Verification items for the finished model (mm, model axes). A direction names the side the tool comes from. Give positions to 0.01 mm unless a question says otherwise; leave off trailing zeros. Write each question's results on one line, items separated by ' | '. Start each with the question number.
1. Material ranges on L1, parallel to Y at x = -57, z = 0.8; L2, parallel to Y at x = 64.5, z = 0.55; L3, parallel to Y at x = -56, z = 0.8, recorded low to high. Write a range as from..to.
2. Cross-section at A-A, the plane z = 0.8. State how many separate pieces and enclosed holes the cut face has, then the cut area to 3 significant figures.
3. Depth check by flat-ended pin: pin 1 Ø0.6 at (y, z) = (5, 0.5) entering from +X; pin 2 Ø0.6 at (y, z) = (14, 0.5) entering from +X; pin 3 Ø0.6 at (x, z) = (2, 1) entering from +Y. Enter the tip coordinate at first touch or a pass-through.
4. Set-up check for faces 4 (the face through (60.76, 30.4, 0.59)), 5 (the face through (31.687, 26.41, 0.592)), 6 (the face through (12.6, 8.6, 0)): record each of +Z, -Z, +X, -X, +Y, -Y from which the full face is reachable in a straight line by a thin tool's end or side.
5. Mould release check, pull along X, two halves, no side actions. Record for faces 1 (the face through (12.6, 8.6, 1.2)), 2 (the face through (61.327, 31.148, 0.592)), 3 (the face through (-42.252, 27.808, 0.592)): +X half, -X half, draft (parallel to the pull), parting line (faces both ways), or undercut.
from build123d import *

# Parameters (mm, degrees)
F1_DEPTH = 1.2


with BuildPart() as f1:
    # F0 (on Top) → F1 (new body)
    with BuildSketch(Plane.XY):
        Polygon((-8.791217, 10.820824), (-8.791217, 15.58735), (-1.791217, 15.58735), (-1.791217, 0), (0, 0), (2.168675, 0), (2.168675, 7.725904), (4.33735, 7.725904), (4.33735, 13.147592), (6.77711, 13.147592), (9.759036, 15.58735), (11.755203, 13.147592), (11.755203, 7.725904), (17.3494, 7.725904), (17.3494, 30.496988), (26.024099, 30.496988), (26.024099, 7.725904), (26.024099, 0), (30.903617, 0), (30.903617, 19.495524), (30.903617, 24.262048), (33.421363, 27.499158), (34.764209, 26.454724), (36.612159, 26.454724), (36.612159, 24.262048), (36.612159, 0), (40.858796, 0), (40.858796, 19.495524), (44.108796, 25.124689), (47.358796, 19.495524), (47.358796, 8.10998), (50.963856, 8.10998), (50.963856, 3.388554), (54.483884, 3.388554), (54.483884, 26.713658), (58.685689, 33.991398), (62.887494, 26.713658), (62.887494, 3.388554), (67.212614, 3.388554), (67.212614, 8.810241), (71.00779, 8.810241), (71.00779, 3.388554), (74.802975, 3.388554), (74.802975, 0), (75.802975, 0), (75.802975, 4.388554), (74.802975, 4.388554), (72.00779, 4.388554), (72.00779, 9.810241), (68.572836, 9.810241), (66.212614, 9.810241), (66.212614, 6.689354), (66.212614, 4.388554), (64.699309, 4.388554), (63.875258, 4.388554), (63.887494, 26.713658), (58.694566, 35.708074), (53.483884, 26.682909), (53.483884, 4.388554), (51.963856, 4.388554), (51.963856, 9.10998), (48.358796, 9.10998), (48.358796, 19.495524), (44.108796, 26.85674), (39.858796, 19.495524), (39.858796, 1), (37.612159, 1), (37.612159, 27.454724), (34.764209, 27.454724), (34.232993, 27.867891), (33.421363, 28.499158), (29.903617, 24.262048), (29.903617, 1), (27.024099, 1), (27.024099, 31.496988), (16.3494, 31.496988), (16.3494, 8.725904), (12.755203, 8.725904), (12.755203, 13.147592), (9.759036, 16.58735), (6.77711, 14.147592), (4.33735, 14.147592), (3.33735, 14.147592), (3.33735, 8.725904), (1.168675, 8.725904), (1.168675, 1), (-0.791217, 1), (-0.791217, 16.58735), (-9.791217, 16.58735), (-9.791217, 11.820824), (-16.291217, 11.820824), (-16.291217, 1), (-21.771085, 1), (-21.771085, 11.820824), (-25.821578, 11.820824), (-25.821578, 20.495524), (-30.47494, 20.495524), (-36.512049, 20.495524), (-36.512049, 1), (-40.204821, 1), (-40.204821, 24.262048), (-44.357452, 31.454616), (-48.510083, 24.262048), (-48.510083, 1), (-55.096389, 1), (-55.096389, 14.208821), (-61.347563, 14.208821), (-61.347563, 16.556969), (-66.283464, 16.556969), (-66.144578, 0), (-65.144543, 0), (-65.275041, 15.556969), (-62.351945, 15.581489), (-62.347563, 15.059114), (-62.347563, 13.208821), (-56.096389, 13.208821), (-56.096389, 0), (-51.847431, 0), (-47.510083, 0), (-47.510083, 24.262048), (-44.357452, 29.722565), (-41.204821, 24.262048), (-41.204821, 0), (-35.512049, 0), (-35.512049, 19.495524), (-26.821578, 19.495524), (-26.821578, 10.820824), (-22.771085, 10.820824), (-22.771085, 0), (-17.891567, 0), (-15.291217, 0), (-15.291217, 1), (-15.291217, 10.820824), align=None)
        Polygon((0, 0), (-1.791217, 0), (-15.291217, 0), (-17.891567, 0), (-22.771085, 0), (-35.512049, 0), (-41.204821, 0), (-47.510083, 0), (-51.847431, 0), (-56.096389, 0), (-65.144543, 0), (-66.144578, 0), (-71.747227, -0.046997), (-71.730845, -2), (74.802975, -2), (75.802975, -2), (75.802975, 0), (74.802975, 0), (40.858796, 0), (36.612159, 0), (30.903617, 0), (26.024099, 0), (2.168675, 0), align=None)
    extrude(amount=F1_DEPTH)


solid = f1.part
Results below:
1) L1: y = -2..0, 13.21..14.21 | L2: y = -2..0, 3.39..4.39 | L3: y = -2..14.21
2) separate pieces: 1 | enclosed holes: 7 | area: 820 mm²
3) pin 1: stops at x = 72.01 | pin 2: stops at x = 63.88 | pin 3: stops at y = 8.73
4) face 4: +Z, -Z | face 5: +Z, -Z, +Y | face 6: -Z, +X, -X, +Y, -Y
5) face 1: draft | face 2: +X half | face 3: undercut
